```python
from build123d import *

# Parameters (mm, degrees)
SKETCH_1_R          = 20
SKETCH_3_R          = 20
SKETCH_3_R_2        = 18.5
EXTRUDE_1_DEPTH     = 15
CUT_EXTRUDE_1_DEPTH = 57.789083564
CUT_EXTRUDE_2_DEPTH = 35


with BuildPart() as part:
    # 扫描1: sweep along a path in 草图2
    with BuildLine(Plane(origin=(0, 0, 0), x_dir=(1, 0, 0), z_dir=(0, 1, 0))) as sweep_1_path:
        ThreePointArc((20, 20), (5.857864376, 14.142135624), (0, 0))
    # 草图1 → 扫描1 (sweep)
    with BuildSketch(Plane.XY):
        Circle(SKETCH_1_R)
    sweep(path=sweep_1_path.line)

    # 草图3 → 凸台-拉伸1 (add)
    with BuildSketch(Plane(origin=(20, 0, 0), x_dir=(0, 0, -1), z_dir=(1, 0, 0))):
        with Locations(Location((20, 0, 0), (0, 0, 180))):
            Circle(SKETCH_3_R)
        with Locations((20, 0)):
            Circle(SKETCH_3_R_2, mode=Mode.SUBTRACT)
    extrude(amount=EXTRUDE_1_DEPTH)

    # 草图4 → 切除-拉伸1 (cut, through all)
    with BuildSketch(Plane.XY):
        with BuildLine():
            Line((-10, 8.25), (-10, 10))
            Line((-10, 10), (-8.25, 10))
            ThreePointArc((-8.25, 10), (-11.237436867, 11.237436867), (-10, 8.25))
        make_face()
        with BuildLine():
            Line((-8.25, 10), (-10, 10))
            Line((-10, 10), (-10, 8.25))
            ThreePointArc((-10, 8.25), (-8.762563133, 8.762563133), (-8.25, 10))
        make_face()
        with BuildLine():
            ThreePointArc((11.75, 10), (10, 11.75), (8.25, 10))
            Line((8.25, 10), (10, 10))
            Line((10, 10), (10, 8.25))
            ThreePointArc((10, 8.25), (11.237436867, 8.762563133), (11.75, 10))
        make_face()
        with BuildLine():
            Line((10, 10), (8.25, 10))
            ThreePointArc((8.25, 10), (8.762563133, 8.762563133), (10, 8.25))
            Line((10, 8.25), (10, 10))
        make_face()
        with BuildLine():
            ThreePointArc((11.75, -10), (11.237436867, -8.762563133), (10, -8.25))
            Line((10, -8.25), (10, -10))
            Line((10, -10), (8.25, -10))
            ThreePointArc((8.25, -10), (10, -11.75), (11.75, -10))
        make_face()
        with BuildLine():
            Line((10, -10), (10, -8.25))
            ThreePointArc((10, -8.25), (8.762563133, -8.762563133), (8.25, -10))
            Line((8.25, -10), (10, -10))
        make_face()
        with BuildLine():
            ThreePointArc((-8.25, -10), (-8.762563133, -8.762563133), (-10, -8.25))
            Line((-10, -8.25), (-10, -10))
            Line((-10, -10), (-8.25, -10))
        make_face()
        with BuildLine():
            Line((-10, -10), (-10, -8.25))
            ThreePointArc((-10, -8.25), (-11.237436867, -11.237436867), (-8.25, -10))
            Line((-8.25, -10), (-10, -10))
        make_face()
    extrude(amount=-CUT_EXTRUDE_1_DEPTH, mode=Mode.SUBTRACT)

    # 草图5 → 切除-拉伸2 (cut)
    with BuildSketch(Plane.XY.offset(-40)):
        with BuildLine():
            ThreePointArc((14, 10), (10, 14), (6, 10))
            Line((6, 10), (10, 10))
            Line((10, 10), (10, 6))
            ThreePointArc((10, 6), (12.828427125, 7.171572875), (14, 10))
        make_face()
        with BuildLine():
            Line((10, 10), (6, 10))
            ThreePointArc((6, 10), (7.171572875, 7.171572875), (10, 6))
            Line((10, 6), (10, 10))
        make_face()
        with BuildLine():
            Line((-10, 6), (-10, 10))
            Line((-10, 10), (-6, 10))
            ThreePointArc((-6, 10), (-12.828427125, 12.828427125), (-10, 6))
        make_face()
        with BuildLine():
            Line((-6, 10), (-10, 10))
            Line((-10, 10), (-10, 6))
            ThreePointArc((-10, 6), (-7.171572875, 7.171572875), (-6, 10))
        make_face()
        with BuildLine():
            ThreePointArc((14, -10), (12.828427125, -7.171572875), (10, -6))
            Line((10, -6), (10, -10))
            Line((10, -10), (6, -10))
            ThreePointArc((6, -10), (10, -14), (14, -10))
        make_face()
        with BuildLine():
            Line((10, -10), (10, -6))
            ThreePointArc((10, -6), (7.171572875, -7.171572875), (6, -10))
            Line((6, -10), (10, -10))
        make_face()
        with BuildLine():
            ThreePointArc((-6, -10), (-7.171572875, -7.171572875), (-10, -6))
            Line((-10, -6), (-10, -10))
            Line((-10, -10), (-6, -10))
        make_face()
        with BuildLine():
            Line((-10, -10), (-10, -6))
            ThreePointArc((-10, -6), (-12.828427125, -12.828427125), (-6, -10))
            Line((-6, -10), (-10, -10))
        make_face()
    extrude(amount=CUT_EXTRUDE_2_DEPTH, mode=Mode.SUBTRACT)


solid = part.part
```
The model under review builds one solid part; all positions refer to its coordinate system, in mm. A direction names the side the tool comes from. Round coordinates to 2 decimals unless told otherwise and drop trailing zeros.
(1) Insertion check: pin 1 (9 mm diameter, centred on x = 9.5, y = 10.5, fed in from -Z); pin 2 (2 mm diameter, centred on y = -9, z = -4.5, fed in from -X); pin 3 (5.5 mm diameter, centred on x = -10, y = 10, fed in from -Z). Each pin has a flat end and moves straight along its axis. Give the tip position at first contact, or say it passes through.
(2) Mouldability with a two-part tool opening along Z and no side actions: class faces 1 (the flat face through (-8, -11, -5)), 2 (the cylindrical face through (27.395, -6.007, -0.924)), 3 (the cylindrical face through (27.4, -18.06, -15.99)) as +Z half, -Z half, draft (parallel to the pull), parting line (faces both ways), or undercut.
(3) Wall thickness on L1, parallel to Y at x = 12.5, z = -32; L2, parallel to Y at x = -10, z = -1.3; L3, parallel to X at y = 10, z = -1.8: over which ranges is each line inside the solid? List them lowest first.
(4) We need section A-A on z = -26. Give the number of separate pieces and of enclosed holes in the cut face, and give its area (3 significant figures).
(5) Machinability: for faces 4 (the flat face through (35, 18, -14)), 5 (the flat face through (11, -12, -5)), 6 (the flat face through (20, 0, -20)), which of the approach directions +Z, -Z, +X, -X, +Y, -Y give a long, thin tool a straight path to every point of the face, cutting with its end or side? Answer none if there is none.
Findings below:
1. pin 1: stops at z = -37.71
1. pin 2: stops at x = -18.08
1. pin 3: stops at z = -5
2. face 1: -Z half
2. face 2: parting line
2. face 3: undercut
3. L1: y = -15.31 to -13.12, -6.88 to 6.88, 13.12 to 15.31
3. L2: y = -17.3 to -11.75, -8.25 to 8.25, 11.75 to 17.3
3. L3: x = -17.28 to -11.75, -8.25 to 8.25, 11.75 to 18.02
4. separate pieces: 1
4. enclosed holes: 2
4. area: 883 mm2
5. face 4: +Z, -Z, +X, +Y, -Y
5. face 5: -Z
5. face 6: +X
